```python
from build123d import *

# Parameters (mm, degrees)
F1_DEPTH = 150


with BuildPart() as f1:
    # F0 (on Top) → F1 (new body)
    with BuildSketch(Plane.XY):
        with BuildLine():
            ThreePointArc((80, 0), (59.9118925632, 302.6549190084), (0, 600))
            Line((0, 600), (0, 0))
            Line((0, 0), (80, 0))
        make_face()
    extrude(amount=F1_DEPTH)

    # F2: F1 across face


with BuildPart() as f1_1:
    add(f1.part)
    add(f1.part.mirror(Plane(origin=(0, 300, 75), x_dir=(0, -1, 0), z_dir=(-1, 0, 0))))

    # F3: F1 across plane


with BuildPart() as f1_2:
    add(f1_1.part)
    add(f1_1.part.mirror(Plane.XZ))


solid = f1_2.part
```
The listing builds one solid part. Answer for the finished solid, in the listing's coordinates (mm). Coordinates: 2 decimals unless noted, no trailing zeros. Write each loop counter-clockwise with the first axis right and the second up, starting at its lowest first coordinate (ties: lowest second). Pieces come first, ordered by that corner, then holes. Notation, with made-up numbers: (5.5, 16) - (18.5, 16) arc R32 cw to (18.5, 43) - close; hole circle Ø4 at (-11, 75). An arc over 180 degrees is marked (long way). Return JSON: item names as keys, results as strings. Group by question number.
Q1. The part is cut by section B-B on y = -206.5. Write down the section's boundary in (x, z).
Q2. Flat-ended cylindrical pins translate along their axes: pin 1 Ø10 at (y, z) = (-287, 124.5) entering from +X; pin 2 Ø2 at (y, z) = (409, 77) entering from +X; pin 3 Ø1.5 at (y, z) = (-325.5, 134) entering from -X. Find the tip coordinate at first contact, or state that the pin passes through.
Q3. The part is cut by section A-A on z = 31. Write down the section's boundary in (x, y).
Q4. Find the intervals of material crossed by line 1 along X through (y, z) = (-396, 69.5); line 2 along X through (y, z) = (248, 81), in increasing order. Write a range as [from, to].
Evaluation:
{
 "1": {"outline": "(-70.67, 0) - (70.67, 0) - (70.67, 150) - (-70.67, 150) - close"},
 "2": {"pin 1": "stops at x = 62.57", "pin 2": "stops at x = 43.36", "pin 3": "stops at x = -56.86"},
 "3": {"outline": "(0, -600) arc R2290 ccw to (0, 600) arc R2290 ccw to start"},
 "4": {"line 1": "x = [-45.5, 45.5]", "line 2": "x = [-66.53, 66.53]"}
}
